```python
from build123d import *

# Parameters (mm, degrees)
F1_DEPTH = 889
F2_W     = 234.95
F2_H     = 171.45
F2_R     = 17.4625
F2_W_2   = 304.8
F3_DEPTH = 25.4
F4_W     = 101.6
F4_H     = 825.5
F4_R     = 14.2875
F5_DEPTH = 25.4
F8_DEPTH = 12.7


with BuildPart() as f1:
    # F0 (on Right) → F1 (new body, symmetric)
    with BuildSketch(Plane.YZ):
        with BuildLine():
            Line((0, 260.35), (-361.95, 260.35))
            ThreePointArc((-361.95, 260.35), (-384.4006403027, 251.0506403027), (-393.7, 228.6))
            Line((-393.7, 228.6), (-393.7, -228.6))
            ThreePointArc((-393.7, -228.6), (-399.2796158184, -242.0703841816), (-412.75, -247.65))
            Line((-412.75, -247.65), (-520.7, -247.65))
            Line((-520.7, -247.65), (-520.7, -260.35))
            Line((-520.7, -260.35), (-412.75, -260.35))
            ThreePointArc((-412.75, -260.35), (-390.2993596973, -251.0506403027), (-381, -228.6))
            Line((-381, -228.6), (-381, 228.6))
            ThreePointArc((-381, 228.6), (-375.4203841816, 242.0703841816), (-361.95, 247.65))
            Line((-361.95, 247.65), (0, 247.65))
            Line((0, 247.65), (361.95, 247.65))
            ThreePointArc((361.95, 247.65), (375.4203841816, 242.0703841816), (381, 228.6))
            Line((381, 228.6), (381, -228.6))
            ThreePointArc((381, -228.6), (390.2993596973, -251.0506403027), (412.75, -260.35))
            Line((412.75, -260.35), (520.7, -260.35))
            Line((520.7, -260.35), (520.7, -247.65))
            Line((520.7, -247.65), (412.75, -247.65))
            ThreePointArc((412.75, -247.65), (399.2796158184, -242.0703841816), (393.7, -228.6))
            Line((393.7, -228.6), (393.7, 228.6))
            ThreePointArc((393.7, 228.6), (384.4006403027, 251.0506403027), (361.95, 260.35))
            Line((361.95, 260.35), (0, 260.35))
        make_face()
    extrude(amount=F1_DEPTH, both=True)

    # F2 (on face) → F3 (join)
    with BuildSketch(Plane.XY.offset(260.35)):
        with Locations((269.875, -269.875)):
            Rectangle(F2_W, F2_H)
        with Locations((279.4, -285.75)):
            Circle(F2_R, mode=Mode.SUBTRACT)
        with Locations((-400.05, -269.875)):
            Rectangle(F2_W_2, F2_H)
        with Locations((-444.5, -285.75)):
            Circle(F2_R, mode=Mode.SUBTRACT)
        with Locations((-400.05, 269.875)):
            Rectangle(F2_W_2, F2_H)
        with Locations((-444.5, 285.75)):
            Circle(F2_R, mode=Mode.SUBTRACT)
        with Locations((269.875, 269.875)):
            Rectangle(F2_W, F2_H)
        with Locations((279.4, 285.75)):
            Circle(F2_R, mode=Mode.SUBTRACT)
    extrude(amount=F3_DEPTH)

    # F4 (on face) → F5 (join)
    with BuildSketch(Plane.XY.offset(260.35)):
        with Locations((473.202, 57.15)):
            Rectangle(F4_W, F4_H)
        with Locations((476.25, -234.95)):
            Circle(F4_R, mode=Mode.SUBTRACT)
        with Locations((476.25, 234.95)):
            Circle(F4_R, mode=Mode.SUBTRACT)
        Polygon((758.698, -355.6), (860.298, -355.6), (860.298, 361.95), (860.298, 469.9), (758.698, 469.9), (758.698, 361.95), align=None)
        with Locations((806.45, -234.95)):
            Circle(F4_R, mode=Mode.SUBTRACT)
        with Locations((806.45, 234.95)):
            Circle(F4_R, mode=Mode.SUBTRACT)
    extrude(amount=F5_DEPTH)

    # F7 (on offset) → F8 (join)
    with BuildSketch(Plane.YZ.offset(711.2)):
        Polygon((-361.95, 247.65), (-381, 228.6), (-381, -247.65), (381, -247.65), (381, 228.6), (361.95, 247.65), align=None)
    extrude(amount=-F8_DEPTH)


solid = f1.part
```
The listing builds one solid part. Answer for the finished solid, in the listing's coordinates (mm). A direction names the side the tool comes from. Coordinates: 2 decimals unless noted, no trailing zeros. Write each loop counter-clockwise with the first axis right and the second up, starting at its lowest first coordinate (ties: lowest second). Pieces come first, ordered by that corner, then holes. Notation, with made-up numbers: (1.25, 88) - (54.25, 88) arc R6 cw to (54.25, 97) - close; hole circle Ø5 at (4.25, 73). An arc over 180 degrees is marked (long way). Return JSON: item names as keys, results as strings. Group by question number.
1. A cutting plane is placed at C-C, the plane z = 192.5. Determine the outline of the cut face in (x, y).
2. A cutting plane is placed at A-A, the plane x = -380. Determine the outline of the cut face in (y, z).
3. Which of the six approach directions +Z, -Z, +X, -X, +Y, -Y give full straight-line access (tool end or side, diameter ignored) to faces 4 (the flat face through (-444, -286, 260.35)), 5 (the flat face through (711.2, -5, 3)), 6 (the flat face through (698.5, -5, 3))?
4. A cutting plane is placed at B-B, the plane y = -80. Determine the outline of the cut face in (x, z).
5. Given pin 1 (10 mm diameter, centred on x = 470, y = -216.5, fed in from -Z); pin 2 (10 mm diameter, centred on x = -403, z = -169, fed in from +Y); pin 3 (1 mm diameter, centred on y = 243, z = -163.5, fed in from +X), each flat-ended and moving along its own axis, determine where each tip first touches the part or whether it passes through.
6. Straight lines are drawn through the part: L1, parallel to X at y = 285, z = 270; L2, parallel to Y at x = -444.5, z = 276.5; L3, parallel to Y at x = 646.5, z = -207. For each, find the intervals that lie inside material, in ascending order.
7. Determine the mould class of faces 1 (the flat face through (12, -467, -260.35)), 2 (the flat face through (12, -393.7, 3)), 3 (the flat face through (280, 286, 260.35)) for opening direction Y: released by +Y, released by -Y, zero draft, split by the parting line, or undercut.
Ans:
{
 "1": {"outline": "(-889, -393.7) - (889, -393.7) - (889, -381) - (711.2, -381) - (711.2, 381) - (889, 381) - (889, 393.7) - (-889, 393.7) - (-889, 381) - (698.5, 381) - (698.5, -381) - (-889, -381) - close"},
 "2": {"outline": "(-520.7, -260.35) - (-412.75, -260.35) arc R31.75 ccw to (-381, -228.6) - (-381, 228.6) arc R19.05 cw to (-361.95, 247.65) - (361.95, 247.65) arc R19.05 cw to (381, 228.6) - (381, -228.6) arc R31.75 ccw to (412.75, -260.35) - (520.7, -260.35) - (520.7, -247.65) - (412.75, -247.65) arc R19.05 cw to (393.7, -228.6) - (393.7, 228.6) arc R31.75 ccw to (361.95, 260.35) - (355.6, 260.35) - (355.6, 285.75) - (184.15, 285.75) - (184.15, 260.35) - (-184.15, 260.35) - (-184.15, 285.75) - (-355.6, 285.75) - (-355.6, 260.35) - (-361.95, 260.35) arc R31.75 ccw to (-393.7, 228.6) - (-393.7, -228.6) arc R19.05 cw to (-412.75, -247.65) - (-520.7, -247.65) - close"},
 "3": {"face 4": "+Z", "face 5": "-Z, +X", "face 6": "-Z, -X"},
 "4": {"outline": "(-889, 247.65) - (698.5, 247.65) - (698.5, -247.65) - (711.2, -247.65) - (711.2, 247.65) - (889, 247.65) - (889, 260.35) - (860.3, 260.35) - (860.3, 285.75) - (758.7, 285.75) - (758.7, 260.35) - (524, 260.35) - (524, 285.75) - (422.4, 285.75) - (422.4, 260.35) - (-889, 260.35) - close"},
 "5": {"pin 1": "z = 247.65", "pin 2": "y = 393.7", "pin 3": "x = 711.2"},
 "6": {"L1": "-552.45 to -461.95, -427.05 to -247.65, 152.4 to 261.95, 296.85 to 387.35, 422.4 to 524, 758.7 to 860.3", "L2": "-355.6 to -303.21, -268.29 to -184.15, 184.15 to 268.29, 303.21 to 355.6", "L3": "-393.7 to -381, 381 to 393.7"},
 "7": {"face 1": "zero draft", "face 2": "released by -Y", "face 3": "undercut"}
}
